from build123d import *

# Parameters (mm, degrees)
BOSS_EXTRUDE1_DEPTH       = 10
CHAMFER1_SIZE             = 3
M3X0_5_TAPPED_HOLE1_D     = 2.5
M3X0_5_TAPPED_HOLE1_DEPTH = 14.5
M3X0_5_TAPPED_HOLE1_TIP   = 0.751075774


with BuildPart() as part:
    # Sketch1 → Boss-Extrude1 (new body)
    with BuildSketch(Plane(origin=(0, 0, 0), x_dir=(0, 0, -1), z_dir=(1, 0, 0))):
        with BuildLine():
            Line((0, 1), (0, 3))
            Line((0, 3), (5, 3))
            Line((5, 3), (5, -10))
            Line((5, -10), (-25.27, -10))
            Line((-25.27, -10), (-25.27, 0))
            Line((-25.27, 0), (-14.5, 0))
            Line((-14.5, 0), (-14.5, -1))
            Line((-14.5, -1), (0, -1))
            ThreePointArc((0, -1), (1, 0), (0, 1))
        make_face()
    extrude(amount=-BOSS_EXTRUDE1_DEPTH)

    # Chamfer1
    chamfer1_edges = [part.edges().sort_by_distance(p)[0] for p in [
        (-5, 3, -5),
        (-5, -10, -5),
    ]]
    chamfer(chamfer1_edges, length=CHAMFER1_SIZE)

    # M3x0.5 Tapped Hole1
    with Locations(Plane(origin=(-5, -5, 25.27), x_dir=(1, 0, 0), z_dir=(0, 0, 1))):
        with Locations((0, 0)):
            Hole(M3X0_5_TAPPED_HOLE1_D / 2, depth=M3X0_5_TAPPED_HOLE1_DEPTH)
            with Locations((0, 0, -(M3X0_5_TAPPED_HOLE1_DEPTH + M3X0_5_TAPPED_HOLE1_TIP / 2))):  # 118° drill point
                Cone(0, M3X0_5_TAPPED_HOLE1_D / 2, M3X0_5_TAPPED_HOLE1_TIP, mode=Mode.SUBTRACT)


solid = part.part
Verification items for the finished model (mm, model axes). A direction names the side the tool comes from. Coordinates: 2 decimals unless noted, no trailing zeros. Order: outer loops, then holes, each group sorted by start corner. A loop starts at its lowest first (then second) coordinate and runs counter-clockwise, first axis right, second up. Notation, with made-up numbers: (-27, 27.5) -> (-23, 27.5) arc R9 cw to (-23, 42.5) -> close; hole circle Ø11 at (-7, 48). An arc over 180 degrees is marked (long way). Put each result on its own line as item: value. Start each with the question number.
1. Material ranges on L1, parallel to Y at x = -5, z = 17; L2, parallel to Y at x = -6.5, z = 10, recorded low to high. Write a range as [from, to].
2. Cross-section at A-A, the plane z = 21. Record the boundary of the cut face in (x, y), then the cut area to 3 significant figures.
3. Go/stop test with flat-tipped pins: pin 1 Ø5 at (x, z) = (-4.5, 0.5) entering from +Y; pin 2 Ø3 at (x, z) = (-5.5, 19.5) entering from +Y; pin 3 Ø2 at (x, y) = (-4.5, 2) entering from +Z. Record where each tip stops, or that it passes through.
4. Cross-section at B-B, the plane x = -7.5. Record the boundary of the cut face in (y, z).
5. Cross-section at D-D, the plane y = -8.25. Record the boundary of the cut face in (x, z).
6. Mould release check, pull along X, two halves, no side actions. Record for faces 1 (the flat face through (-10, -5, 10)), 2 (the flat face through (-5, -10, 11)), 3 (the cylindrical face through (-4.73, -6.22, 17.92)): released by +X, released by -X, zero draft, split by the parting line, or undercut.
7. Access from +Z, -Z, +X, -X, +Y, -Y to the whole of each face (thin tool, end or side, straight path). Record for faces 4 (the flat face through (-5, 0, 20)), 5 (the flat face through (-4.9, -0.5, 14.5)), 6 (the cylindrical face through (-5, 0, -1)).
8. Cross-section at C-C, the plane y = 1.75. Record the boundary of the cut face in (x, z).
Computed:
1. L1: [-10, -6.25], [-3.75, 0]
1. L2: [-10, -1]
2. outline: (-10, -10) -> (0, -10) -> (0, 0) -> (-10, 0) -> close; hole circle Ø2.5 at (-5, -5)
2. area: 95.1 mm2
3. pin 1: y = 3
3. pin 2: y = 0
3. pin 3: z = 0
4. outline: (-10, -2) -> (-7, -5) -> (0, -5) -> (3, -2) -> (3, 0) -> (1, 0) arc R1 cw to (-1, 0) -> (-1, 14.5) -> (0, 14.5) -> (0, 25.27) -> (-10, 25.27) -> close
5. outline: (-10, -3.75) -> (0, -3.75) -> (0, 25.27) -> (-10, 25.27) -> close
6. face 1: released by -X
6. face 2: zero draft
6. face 3: undercut
7. face 4: +Z, +X, -X, +Y
7. face 5: +X, -X, +Y
7. face 6: +X, -X
8. outline: (-10, -3.25) -> (0, -3.25) -> (0, 0) -> (-10, 0) -> close
